Source: CAD feature listing. Evaluate the final solid. Frame: model axes, mm. Face numbers are marked on the shaded views. A direction names the side the tool comes from. Round coordinates to 2 decimals unless told otherwise and drop trailing zeros. Order: outer loops, then holes, each group sorted by start corner. A loop starts at its lowest first (then second) coordinate and runs counter-clockwise, first axis right, second up. Notation, with made-up numbers: (67.5, 34.25) - (82.5, 34.25) arc R7 cw to (82.5, 45.25) - close; hole circle Ø9 at (-4.5, -26). An arc over 180 degrees is marked (long way). Return JSON: item names as keys, results as strings. Group by question number.
1) Section C-C, the plane z = 6. Return loops of the section in (x, y) (3 decimals), plus the area to 3 significant figures.
2) Access query for the marked faces 3 and 4. Directions: +Z, -Z, +X, -X, +Y, -Y. A direction counts if a zero-diameter tool reaches every point of the face in a straight line with its end or side. Return the directions, or none.
3) Section D-D, the plane x = 14.5. Return loops of the section in (y, z).
4) Section A-A, the plane y = 24. Return loops of the section in (x, z).
5) Contact query for flat-ended pins moving along their axis: P1, Ø4, axis at y = 50, z = 11, coming from the +X side; P2, Ø2, axis at x = 10, z = 8.5, coming from the +Y side; P3, Ø15, axis at x = 44.14, y = 54.13, coming from the -Z side; P4, Ø6, axis at x = 22, z = 6.5, coming from the +Y side. Output: stop coordinate, or through.
6) Ray query, line 1 (Y direction, x = 45, z = 2); line 2 (Y direction, x = 35.5, z = 10.25); line 3 (X direction, y = 14, z = 6.5). Return the intervals inside material, ascending. Write a range as from..to.
7) Mould query, pull axis X, two halves, no side actions, for the marked faces 1 and 2. Classes: pulls with the +X half, pulls with the -X half, needs draft (parallel to the pull), parting line crosses it, or undercut.
8) Section B-B, the plane x = 45. Return loops of the section in (y, z), plus the area to 3 significant figures.
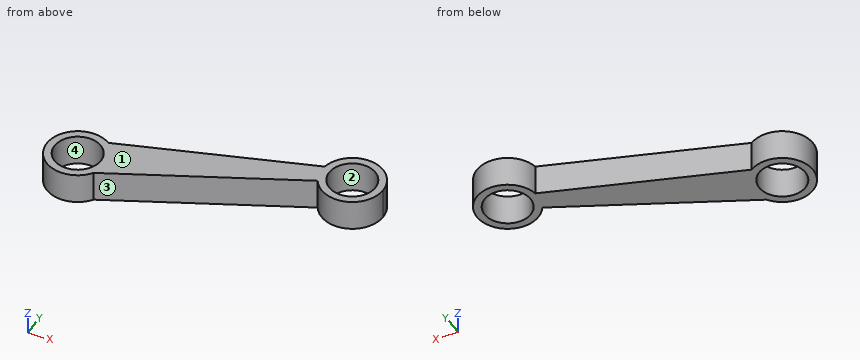
```python
from build123d import *

# Parameters (mm, degrees)
F1_DEPTH = 12.7
F3_D     = 19.05


with BuildPart() as f1:
    # F0 (on Top) → F1 (new body)
    with BuildSketch(Plane.XY):
        with BuildLine():
            ThreePointArc((-41.224553, 13.086214), (-39.543115, 16.529238), (-38.965097, 20.317053))
            ThreePointArc((-38.965097, 20.317053), (-40.460249, 26.295463), (-44.593661, 30.866214))
            ThreePointArc((-44.593661, 30.866214), (-64.143057, 17.952622), (-41.224553, 13.086214))
        make_face()
        with BuildLine():
            ThreePointArc((-44.593661, 30.866214), (-40.460249, 26.295463), (-38.965097, 20.317053))
            ThreePointArc((-38.965097, 20.317053), (-39.543115, 16.529238), (-41.224553, 13.086214))
            Line((-41.224553, 13.086214), (33.170466, 47.735668))
            ThreePointArc((33.170466, 47.735668), (31.656753, 51.811239), (31.606339, 56.158545))
            Line((31.606339, 56.158545), (-44.593661, 30.866214))
        make_face()
        with BuildLine():
            ThreePointArc((56.843282, 54.129986), (45.160833, 66.789156), (31.606339, 56.158545))
            ThreePointArc((31.606339, 56.158545), (31.656753, 51.811239), (33.170466, 47.735668))
            ThreePointArc((33.170466, 47.735668), (47.455021, 41.869383), (56.843282, 54.129986))
        make_face()
    extrude(amount=F1_DEPTH)

    # F3 (through all)
    with Locations(Plane.XY.offset(12.7)):
        with Locations((-51.665097, 20.317053), (44.143282, 54.129986)):
            Hole(F3_D / 2)


solid = f1.part
```
Geometry check:
{
 "1": {"outline": "(-44.594, 30.866) arc R12.7 ccw (long way) to (-41.225, 13.086) - (33.17, 47.736) arc R12.7 ccw (long way) to (31.606, 56.159) - close; hole circle Ø19.05 at (-51.665, 20.317); hole circle Ø19.05 at (44.143, 54.13)", "area": "1,450 mm2"},
 "2": {"face 3": "+Z, -Z, -Y", "face 4": "+Z, -Z"},
 "3": {"outline": "(39.04, 0) - (50.48, 0) - (50.48, 12.7) - (39.04, 12.7) - close"},
 "4": {"outline": "(-63.82, 0) - (-60.45, 0) - (-60.45, 12.7) - (-63.82, 12.7) - close; (-42.88, 0) - (-17.79, 0) - (-17.79, 12.7) - (-42.88, 12.7) - close"},
 "5": {"P1": "x = 56.66", "P2": "y = 49.32", "P3": "through", "P4": "y = 53.97"},
 "6": {"line 1": "41.46..44.64, 63.62..66.8", "line 2": "44.82..50.13, 58.13..63.44", "line 3": "-62.68..-58.79, -44.54..-39.26"},
 "7": {"face 1": "needs draft", "face 2": "undercut"},
 "8": {"outline": "(41.46, 0) - (44.64, 0) - (44.64, 12.7) - (41.46, 12.7) - close; (63.62, 0) - (66.8, 0) - (66.8, 12.7) - (63.62, 12.7) - close", "area": "80.9 mm2"}
}
